from build123d import *

# Parameters (mm, degrees)
F1_DEPTH = 60
F2_DEPTH = 25
F0_W     = 105.667732
F0_H     = 72.615263
F0_R     = 11.419882
F0_R_2   = 13.662159
F0_R_3   = 9.028208
F0_R_4   = 12.522377
F0_R_5   = 11.895855
F3_DEPTH = 10
F0_R_6   = 1.784712
F4_DEPTH = 50
F5_DEPTH = 25
F6_DEPTH = 25


with BuildPart() as f1:
    # F0 (on Top) → F1 (new body)
    with BuildSketch(Plane.XY):
        Polygon((-9.727011, 17.693468), (-13.396265, 21.534182), (-15.313769, 16.580629), (-16.401034, 13.77186), (-10.718366, 0), (0, 7.511924), align=None)
    extrude(amount=F1_DEPTH)

    # F0 (on Top) → F2 (join)
    with BuildSketch(Plane.XY):
        with BuildLine():
            Line((-15.313769, 16.580629), (-13.396265, 21.534182))
            Line((-13.396265, 21.534182), (-9.727011, 17.693468))
            ThreePointArc((-9.727011, 17.693468), (-14.433935, 26.743573), (-15.313769, 16.580629))
        make_face()
    extrude(amount=F2_DEPTH)

    # F0 (on Top) → F3 (join)
    with BuildSketch(Plane.XY):
        with Locations((7.88752, 4.757551)):
            Rectangle(F0_W, F0_H)
        with Locations((-30.423293, -4.256757)):
            Circle(F0_R, mode=Mode.SUBTRACT)
        with Locations((23.412162, -14.77345)):
            Circle(F0_R_2, mode=Mode.SUBTRACT)
        with BuildLine():
            Line((-16.401034, 13.77186), (-15.313769, 16.580629))
            ThreePointArc((-15.313769, 16.580629), (-14.433935, 26.743573), (-9.727011, 17.693468))
            Line((-9.727011, 17.693468), (0, 7.511924))
            Line((0, 7.511924), (-10.718366, 0))
            Line((-10.718366, 0), (-16.401034, 13.77186))
        make_face(mode=Mode.SUBTRACT)
        with Locations((-32.676868, 29.5469)):
            Circle(F0_R_3, mode=Mode.SUBTRACT)
        with Locations((41.440781, 5.759142)):
            Circle(F0_R_4, mode=Mode.SUBTRACT)
        with Locations((13.89706, 26.792528)):
            Circle(F0_R_5, mode=Mode.SUBTRACT)
    extrude(amount=F3_DEPTH)

    # F0 (on Top) → F4 (join)
    with BuildSketch(Plane.XY):
        with Locations((13.89706, 26.792528)):
            Circle(F0_R_5)
        with Locations((6.595331, 27.143202)):
            Circle(F0_R_6, mode=Mode.SUBTRACT)
        with Locations((10.773938, 20.183116)):
            Circle(F0_R_6, mode=Mode.SUBTRACT)
        with Locations((18.716843, 21.296355)):
            Circle(F0_R_6, mode=Mode.SUBTRACT)
        with Locations((21.027262, 28.404499)):
            Circle(F0_R_6, mode=Mode.SUBTRACT)
        with Locations((13.482664, 34.090918)):
            Circle(F0_R_6, mode=Mode.SUBTRACT)
        with Locations((13.482664, 34.090918)):
            Circle(F0_R_6)
        with Locations((6.595331, 27.143202)):
            Circle(F0_R_6)
        with Locations((10.773938, 20.183116)):
            Circle(F0_R_6)
        with Locations((18.716843, 21.296355)):
            Circle(F0_R_6)
        with Locations((21.027262, 28.404499)):
            Circle(F0_R_6)
    extrude(amount=F4_DEPTH)

    # F0 (on Top) → F5 (join)
    with BuildSketch(Plane.XY):
        with Locations((10.773938, 20.183116)):
            Circle(F0_R_6)
    extrude(amount=-F5_DEPTH)

    # F0 (on Top) → F6 (cut)
    with BuildSketch(Plane.XY):
        with Locations((21.027262, 28.404499)):
            Circle(F0_R_6)
    extrude(amount=F6_DEPTH, mode=Mode.SUBTRACT)


solid = f1.part
Verification items for the finished model (mm, model axes). A direction names the side the tool comes from. Give positions to 0.01 mm unless a question says otherwise; leave off trailing zeros. Order: outer loops, then holes, each group sorted by start corner. A loop starts at its lowest first (then second) coordinate and runs counter-clockwise, first axis right, second up. Notation, with made-up numbers: M -39.75,69.25 L -35.75,69.25 A18 cw -35.75,89.25 Z; hole C 26.25,86 d5. An arc over 180 degrees is marked long. Answer as a JSON object with one key per item and string values. Group by question number.
1) Cross-section at A-A (y = -9.5). Enter the section's corners in (x, z).
2) Depth check by flat-ended pin: pin 1 Ø1.1 at (x, y) = (21, 28) entering from -Z; pin 2 Ø6 at (y, z) = (25.5, 41) entering from -X; pin 3 Ø6 at (x, y) = (11.5, 28) entering from -Z; pin 4 Ø20 at (x, y) = (41.44, 5.76) entering from -Z. Enter the tip coordinate at first touch or a pass-through.
3) Access from +Z, -Z, +X, -X, +Y, -Y to the whole of each face (thin tool, end or side, straight path). Record for faces 1 (the face through (-13.6, 6.98, 34.65)), 2 (the face through (-14.245, 26.778, 17.395)), 3 (the face through (-5.434, 3.703, 34.65)), 4 (the face through (20.795, 30.174, 12.325)).
4) Mould release check, pull along Y, two halves, no side actions. Record for faces 5 (the face through (5.1, 34.8, 29.7)), 6 (the face through (-10, 11, 60)), 7 (the face through (21, 28, 25)): released by +Y, released by -Y, zero draft, split by the parting line, or undercut.
5) Scan lines: line 1 along X through (y, z) = (3, 0.5); line 2 along Z through (x, y) = (50.5, 21); line 3 along X through (y, z) = (21, 41). Record each from-to range of solid material in increasing order. Write a range as [from, to].
6) Cross-section at B-B (z = 39.5). Enter the section's corners in (x, y), then the cut area to 3 significant figures.
7) Cross-section at C-C (x = -21). Enter the section's corners in (y, z), then the cut area to 3 significant figures.
8) Cross-section at D-D (x = 35). Enter the section's corners in (y, z), then the cut area to 3 significant figures.
Result sheet:
{
 "1": {"outline": "M -44.95,0 L -40.57,0 L -40.57,10 L -44.95,10 Z; M -20.28,0 L 10.81,0 L 10.81,10 L -20.28,10 Z; M 36.02,0 L 60.72,0 L 60.72,10 L 36.02,10 Z"},
 "2": {"pin 1": "stops at z = 25", "pin 2": "stops at x = 2", "pin 3": "stops at z = 0", "pin 4": "passes through"},
 "3": {"face 1": "+Z, -X, -Y", "face 2": "+Z", "face 3": "+Z, +X, -Y", "face 4": "-Z"},
 "4": {"face 5": "split by the parting line", "face 6": "zero draft", "face 7": "undercut"},
 "5": {"line 1": "x = [-44.95, -39.24], [-21.61, 29.23], [53.66, 60.72]", "line 2": "z = [0, 10]", "line 3": "x = [-13.6, -12.89], [3.51, 24.29]"},
 "6": {"outline": "M -16.4,13.77 L -10.72,0 L 0,7.51 L -13.4,21.53 Z; C 13.9,26.79 d23.79", "area": "613 mm2"},
 "7": {"outline": "M -31.55,0 L -10.71,0 L -10.71,10 L -31.55,10 Z; M 2.19,0 L 41.07,0 L 41.07,10 L 2.19,10 Z", "area": "597 mm2"},
 "8": {"outline": "M -31.55,0 L -22.01,0 L -22.01,10 L -31.55,10 Z; M -7.54,0 L -4.98,0 L -4.98,10 L -7.54,10 Z; M 16.5,0 L 41.07,0 L 41.07,10 L 16.5,10 Z", "area": "367 mm2"}
}
